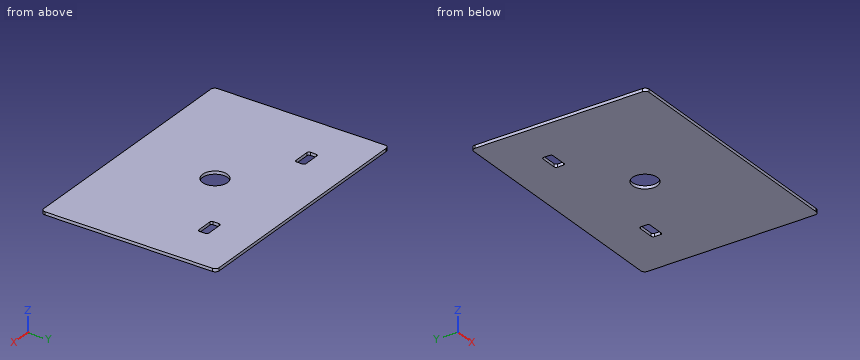
from build123d import *

# Parameters (mm, degrees)
SKETCH1_W           = 252
SKETCH1_H           = 176
BOSS_EXTRUDE1_DEPTH = 3
SKETCH2_R           = 12.5
SKETCH2_W           = 20
SKETCH2_H           = 10
CUT_EXTRUDE1_DEPTH  = 4
FILLET2_R           = 2
FILLET3_R           = 4


with BuildPart() as part:
    # Sketch1 → Boss-Extrude1 (new body)
    with BuildSketch(Plane.XY):
        Rectangle(SKETCH1_W, SKETCH1_H)
    extrude(amount=BOSS_EXTRUDE1_DEPTH)

    # Sketch2 → Cut-Extrude1 (cut, through all)
    with BuildSketch(Plane.XY.offset(3)):
        Circle(SKETCH2_R)
        with Locations((-71, 43)):
            Rectangle(SKETCH2_W, SKETCH2_H)
        with Locations((71, 43)):
            Rectangle(SKETCH2_W, SKETCH2_H)
    extrude(amount=-CUT_EXTRUDE1_DEPTH, mode=Mode.SUBTRACT)

    # Fillet2
    fillet2_edges = [part.edges().sort_by_distance(p)[0] for p in [
        (-81, 38, 1.5),
        (-81, 48, 1.5),
        (-61, 48, 1.5),
        (-61, 38, 1.5),
        (81, 48, 1.5),
        (81, 38, 1.5),
        (61, 38, 1.5),
        (61, 48, 1.5),
    ]]
    fillet(fillet2_edges, radius=FILLET2_R)

    # Fillet3
    fillet3_edges = [part.edges().sort_by_distance(p)[0] for p in [
        (126, -88, 1.5),
        (-126, -88, 1.5),
        (-126, 88, 1.5),
        (126, 88, 1.5),
    ]]
    fillet(fillet3_edges, radius=FILLET3_R)


solid = part.part
Can you work these out from the model? Positions are in its coordinate system, mm. Coordinates: 2 decimals unless noted, no trailing zeros. Write each loop counter-clockwise with the first axis right and the second up, starting at its lowest first coordinate (ties: lowest second). Pieces come first, ordered by that corner, then holes. Notation, with made-up numbers: M 66,6.25 L 90,6.25 A21 ccw 90,39.25 Z; hole C -18.75,87.25 d4. An arc over 180 degrees is marked long. Use one line per item in the form item = value.
Q1. If we section it at C-C (z = 1.8): Write out the boundary of the cut face in (x, y).
Model answer:
outline = M -126,-84 A4 ccw -122,-88 L 122,-88 A4 ccw 126,-84 L 126,84 A4 ccw 122,88 L -122,88 A4 ccw -126,84 Z; hole M -81,40 A2 ccw -79,38 L -63,38 A2 ccw -61,40 L -61,46 A2 ccw -63,48 L -79,48 A2 ccw -81,46 Z; hole C 0,0 d25; hole M 61,40 A2 ccw 63,38 L 79,38 A2 ccw 81,40 L 81,46 A2 ccw 79,48 L 63,48 A2 ccw 61,46 Z
Q2. If we section it at A-A (x = -0.5): Write out the boundary of the cut face in (y, z), then the cut area to 3 significant figures.
Model answer:
outline = M -88,0 L -12.49,0 L -12.49,3 L -88,3 Z; M 12.49,0 L 88,0 L 88,3 L 12.49,3 Z
area = 453 mm^2
Q3. If we section it at B-B (y = 43.5): Write out the boundary of the cut face in (x, z).
Model answer:
outline = M -126,0 L -81,0 L -81,3 L -126,3 Z; M -61,0 L 61,0 L 61,3 L -61,3 Z; M 81,0 L 126,0 L 126,3 L 81,3 Z
Q4. I need wall thicknesses on line 1 along Y through (x, z) = (78, 0.5); line 2 along Y through (x, z) = (0, 1.75); line 3 along X through (y, z) = (8, 1.05). Which ranges of each line are inside material? Lowest first, please. Write a range as from..to.
Model answer:
line_1 = -88..38, 48..88
line_2 = -88..-12.5, 12.5..88
line_3 = -126..-9.6, 9.6..126
Q5. If we section it at D-D (y = 0): Write out the boundary of the cut face in (x, z), then the cut area to 3 significant figures.
Model answer:
outline = M -126,0 L -12.5,0 L -12.5,3 L -126,3 Z; M 12.5,0 L 126,0 L 126,3 L 12.5,3 Z
area = 681 mm^2
Q6. For P1, Ø20, axis at x = 0, y = 0, coming from the +Z side, with a flat end and sliding along its axis, tell me the tip position at first contact or that it passes through.
Model answer:
P1 = through
